Verification items for this drawing (mm, ordinates from the low corner). A direction names the side the tool comes from. Coordinates: 2 decimals unless noted, no trailing zeros. Order: outer loops, then holes, each group sorted by start corner. A loop starts at its lowest first (then second) coordinate and runs counter-clockwise, first axis right, second up. Notation, with made-up numbers: (-27.5, -35.5) -> (15.5, -35.5) arc R7 ccw to (15.5, -24.5) -> close; hole circle Ø7 at (60.25, 0). An arc over 180 degrees is marked (long way). Put each result on its own line as item: value. Start each with the question number.
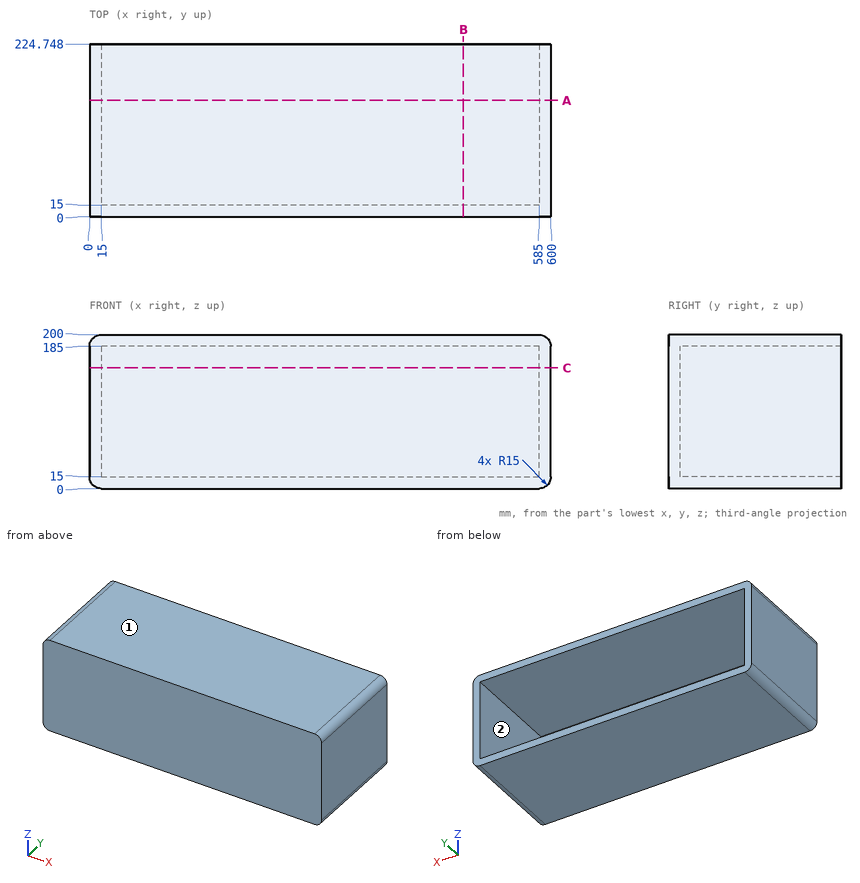
1) Access from +Z, -Z, +X, -X, +Y, -Y to the whole of each face (thin tool, end or side, straight path). Record for the marked faces 1 and 2.
2) Gauge pin test, flat ends, axial feed: pin 1 (4 mm diameter, centred on y = 67, z = 75, fed in from -X); pin 2 (12 mm diameter, centred on x = 253.5, z = 87.5, fed in from +Y). Record the tip position at first contact, or that the pin passes through.
3) Sectioned sample at B-B (x = 486.5). Record the boundary of the cut face in (y, z), plus the area to 3 significant figures.
4) Sectioned sample at C-C (z = 157). Record the boundary of the cut face in (x, y).
5) Sectioned sample at A-A (y = 151.5). Record the boundary of the cut face in (x, z).
6) Scan lines: line 1 along X through (y, z) = (200, 31.5); line 2 along Z through (x, y) = (263, 106.5); line 3 along Y through (x, z) = (143, 19). Record each from-to range of solid material in increasing order. Write a range as [from, to].
Entries:
1. face 1: +Z, +X, -X, +Y, -Y
1. face 2: +Y
2. pin 1: stops at x = 0
2. pin 2: stops at y = 15
3. outline: (0, 0) -> (224.75, 0) -> (224.75, 15) -> (15, 15) -> (15, 185) -> (224.75, 185) -> (224.75, 200) -> (0, 200) -> close
3. area: 9,290 mm2
4. outline: (0, 0) -> (600, 0) -> (600, 224.75) -> (585, 224.75) -> (585, 15) -> (15, 15) -> (15, 224.75) -> (0, 224.75) -> close
5. outline: (0, 15) arc R15 ccw to (15, 0) -> (585, 0) arc R15 ccw to (600, 15) -> (600, 185) arc R15 ccw to (585, 200) -> (15, 200) arc R15 ccw to (0, 185) -> close; hole (15, 15) -> (585, 15) -> (585, 185) -> (15, 185) -> close
6. line 1: x = [0, 15], [585, 600]
6. line 2: z = [0, 15], [185, 200]
6. line 3: y = [0, 15]
